Could you check a few things on this model? Use its own coordinates, in mm. A direction names the side the tool comes from. Give positions to 0.01 mm unless a question says otherwise; leave off trailing zeros. Order: outer loops, then holes, each group sorted by start corner. A loop starts at its lowest first (then second) coordinate and runs counter-clockwise, first axis right, second up. Notation, with made-up numbers: (-36.75, 46.5) -> (-19.75, 46.5) arc R22 cw to (-19.75, 56.5) -> close; hole circle Ø8 at (51.5, 6.5). An arc over 180 degrees is marked (long way). Use one line per item in the form item = value. Start each with the question number.
from build123d import *

# Parameters (mm, degrees)
ESQUISSE1_W             = 200
ESQUISSE1_H             = 100
BOSS_EXTRU_1_DEPTH      = 100
CHANFREIN1_SIZE         = 40
ESQUISSE2_R             = 6.5
ENL_V_MAT_EXTRU_1_DEPTH = 230.128784748
ESQUISSE4_R             = 1.5
ENL_V_MAT_EXTRU_3_DEPTH = 151
ESQUISSE5_W             = 152
ESQUISSE5_H             = 92
ENL_V_MAT_EXTRU_4_DEPTH = 70


with BuildPart() as part:
    # Esquisse1 → Boss.-Extru.1 (new body)
    with BuildSketch(Plane.XY):
        Rectangle(ESQUISSE1_W, ESQUISSE1_H)
    extrude(amount=BOSS_EXTRU_1_DEPTH)

    # Chanfrein1
    chanfrein1_edges = [part.edges().sort_by_distance(p)[0] for p in [
        (-100, -50, 50),
    ]]
    chamfer(chanfrein1_edges, length=CHANFREIN1_SIZE)

    # Esquisse2 → Enlèv. mat.-Extru.1 (cut, through all)
    with BuildSketch(Plane(origin=(100, 0, 0), x_dir=(0, 0, -1), z_dir=(1, 0, 0))):
        with Locations((-50, 30)):
            Circle(ESQUISSE2_R)
    extrude(amount=-ENL_V_MAT_EXTRU_1_DEPTH, mode=Mode.SUBTRACT)

    # Esquisse4 → Enlèv. mat.-Extru.3 (cut, through all)
    with BuildSketch(Plane.XY.offset(100)):
        with Locations((90, -45)):
            Circle(ESQUISSE4_R)
        with Locations((-40, -45)):
            Circle(ESQUISSE4_R)
    extrude(amount=-ENL_V_MAT_EXTRU_3_DEPTH, mode=Mode.SUBTRACT)

    # Esquisse5 → Enlèv. mat.-Extru.4 (cut)
    with BuildSketch(Plane.XZ.offset(50)):
        with Locations((20, 50)):
            Rectangle(ESQUISSE5_W, ESQUISSE5_H)
    extrude(amount=-ENL_V_MAT_EXTRU_4_DEPTH, mode=Mode.SUBTRACT)


solid = part.part
(1) Imagine slicing it at A-A (y = -4.5). Write out the boundary of the cut face in (x, z), plus the area to 3 significant figures.
(2) Imagine slicing it at B-B (z = 68). Write out the boundary of the cut face in (x, y), plus the area to 3 significant figures.
(3) Imagine slicing it at D-D (z = 50). Write out the boundary of the cut face in (x, y), plus the area to 3 significant figures.
(4) Imagine slicing it at C-C (x = -18.5). Write out the boundary of the cut face in (y, z).
(5) Which directions (+Z, -Z, +X, -X, +Y, -Y) give clear straight access to the entire face, cutting with the end or side of a thin tool? Please do faces 1 (the flat face through (19, 20, 51)), 2 (the cylindrical face through (1.4, 34.393, 54.791)).
(6) I'm going to push flat-ended pins straight in: pin 1 Ø10 at (x, y) = (7.5, 16) entering from -Z; pin 2 Ø8 at (y, z) = (30, 50) entering from -X; pin 3 Ø8 at (x, z) = (-48.5, 14) entering from -Y; pin 4 Ø1.5 at (y, z) = (-35.5, 29.5) entering from -X. Where does each tip first touch, or does it pass through?
(7) Please list where these lines run through material, in increasing order: probe 1 along Y at (x, z) = (-40, 98.9); probe 2 along X at (y, z) = (-8.5, 5); probe 3 along Z at (x, y) = (44.5, -36).
(8) We'd pull the mould along Z, two halves only. Please class faces 3 (the flat face through (-1, 1, 0)), 4 (the flat face through (100, -1, 49)), 5 (the flat face through (19, -15, 96)), 6 (the flat face through (-1, 1, 100)): pulls with the +Z half, pulls with the -Z half, needs draft (parallel to the pull), parting line crosses it, or undercut.
Calculated:
q1.outline = (-100, 0) -> (100, 0) -> (100, 100) -> (-100, 100) -> close; hole (-56, 4) -> (96, 4) -> (96, 96) -> (-56, 96) -> close
q1.area = 6,020 mm2
q2.outline = (-100, -10) -> (-60, -50) -> (-56, -50) -> (-56, 20) -> (96, 20) -> (96, -50) -> (100, -50) -> (100, 50) -> (-100, 50) -> close
q2.area = 8,560 mm2
q3.outline = (-100, -10) -> (-60, -50) -> (-56, -50) -> (-56, 20) -> (96, 20) -> (96, -50) -> (100, -50) -> (100, 23.5) -> (-100, 23.5) -> close; (-100, 36.5) -> (100, 36.5) -> (100, 50) -> (-100, 50) -> close
q3.area = 5,960 mm2
q4.outline = (-50, 0) -> (50, 0) -> (50, 100) -> (-50, 100) -> (-50, 96) -> (20, 96) -> (20, 4) -> (-50, 4) -> close; hole circle Ø13 at (30, 50)
q5.face_1 = -Y
q5.face_2 = +X, -X
q6.pin_1 = 0
q6.pin_2 = through
q6.pin_3 = 20
q6.pin_4 = -75.25
q7.probe_1 = -50 to -46.5, -43.5 to 50
q7.probe_2 = -100 to -56, 96 to 100
q7.probe_3 = 0 to 4, 96 to 100
q8.face_3 = pulls with the -Z half
q8.face_4 = needs draft
q8.face_5 = undercut
q8.face_6 = pulls with the +Z half
